Design review of the part built by this model. Coordinates are the model's own, in mm. Face numbers are marked on the shaded views. A direction names the side the tool comes from. Round coordinates to 2 decimals unless told otherwise and drop trailing zeros. Order: outer loops, then holes, each group sorted by start corner. A loop starts at its lowest first (then second) coordinate and runs counter-clockwise, first axis right, second up.
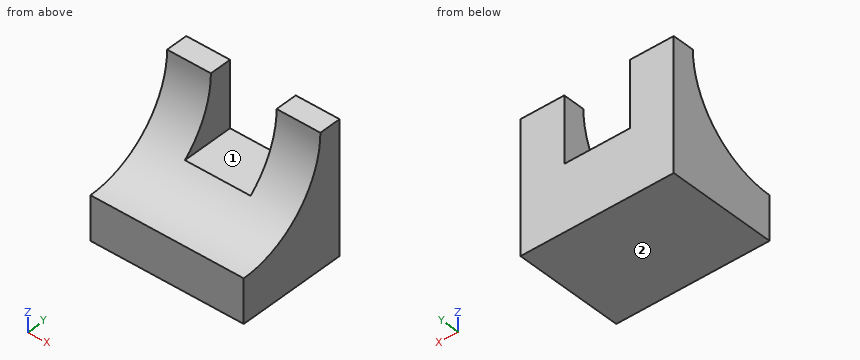
from build123d import *

# Parameters (mm, degrees)
F0_W     = 88.9
F0_H     = 76.2
F1_DEPTH = 63.5
F2_W     = 38.1
F2_H     = 38.1
F3_DEPTH = 63.501
F5_DEPTH = 88.901


with BuildPart() as f1:
    # F0 (on Front) → F1 (new body)
    with BuildSketch(Plane.XZ):
        with Locations((2.397262, -13.328955)):
            Rectangle(F0_W, F0_H)
    extrude(amount=F1_DEPTH)

    # F2 (on face) → F3 (cut, through all)
    with BuildSketch(Plane(origin=(0, 0, 0), x_dir=(-1, 0, 0), z_dir=(0, 1, 0))):
        with Locations((-2.397262, 5.721045)):
            Rectangle(F2_W, F2_H)
    extrude(amount=-F3_DEPTH, mode=Mode.SUBTRACT)

    # F4 (on face) → F5 (cut, through all)
    with BuildSketch(Plane(origin=(-42.052738, 0, 0), x_dir=(0, -1, 0), z_dir=(-1, 0, 0))):
        with BuildLine():
            Line((63.5, 24.771045), (12.7, 24.771045))
            ThreePointArc((12.7, 24.771045), (27.578976, -11.149979), (63.5, -26.028955))
            Line((63.5, -26.028955), (63.5, 24.771045))
        make_face()
    extrude(amount=-F5_DEPTH, mode=Mode.SUBTRACT)


solid = f1.part
1) Take a section at B-B on y = -5.5. Give the boundary of the cut face in (x, z), plus the area to 3 significant figures.
Results:
outline: (-42.05, -51.43) - (46.85, -51.43) - (46.85, 24.77) - (21.45, 24.77) - (21.45, -13.33) - (-16.65, -13.33) - (-16.65, 24.77) - (-42.05, 24.77) - close
area: 5,320 mm2
2) Take a section at A-A on z = 10. Give the boundary of the cut face in (x, y), plus the area to 3 significant figures.
Results:
outline: (-42.05, -14.89) - (-16.65, -14.89) - (-16.65, 0) - (-42.05, 0) - close; (21.45, -14.89) - (46.85, -14.89) - (46.85, 0) - (21.45, 0) - close
area: 757 mm2
3) Take a section at C-C on x = -6.5. Give the boundary of the cut face in (y, z), plus the area to 3 significant figures.
Results:
outline: (-63.5, -51.43) - (0, -51.43) - (0, -13.33) - (-29.9, -13.33) arc R50.8 cw to (-63.5, -26.03) - close
area: 2,130 mm2
4) Take a section at D-D on z = -8.5. Give the boundary of the cut face in (x, y), plus the area to 3 significant figures.
Results:
outline: (-42.05, -25.11) - (-16.65, -25.11) - (-16.65, 0) - (-42.05, 0) - close; (21.45, -25.11) - (46.85, -25.11) - (46.85, 0) - (21.45, 0) - close
area: 1,280 mm2
5) To check wall thickness, follow line 1 along X through (y, z) = (-16, -6); line 2 along Z through (x, y) = (-8.5, -25.5); line 3 along Y through (x, z) = (30, 4.5). State the ranges of each line that lie inside material, in increasing order.
Results:
line 1: x = -42.05 to -16.65, 21.45 to 46.85
line 2: z = -51.43 to -13.33
line 3: y = -16.92 to 0
6) For the marked faces 1 and 2, list the 3-axis set-ups (+Z, -Z, +X, -X, +Y, -Y) from which the entire face can be reached by the end or side of a thin tool; tool diameter is ignored.
Results:
face 1: +Z, +Y, -Y
face 2: -Z, +X, -X, +Y, -Y
7) Clearance check with flat-ended pins moving along their axes: P1, Ø2, axis at x = -15, z = 10.5, coming from the +Y side; P2, Ø24, axis at x = 0, y = -12, coming from the +Z side; P3, Ø4, axis at x = 6.5, z = -16.5, coming from the -Y side; P4, Ø1.5, axis at x = -25.5, z = -6.5, coming from the -Y side. State where each tip first meets the part, or that it passes through.
Results:
P1: passes through
P2: stops at z = -13.33
P3: stops at y = -36.89
P4: stops at y = -24.06
